Can you work these out from the model? Positions are in its coordinate system, mm. Coordinates: 2 decimals unless noted, no trailing zeros. Order: outer loops, then holes, each group sorted by start corner. A loop starts at its lowest first (then second) coordinate and runs counter-clockwise, first axis right, second up. Notation, with made-up numbers: (7, 73) -> (30, 73) arc R11 ccw to (30, 84) -> close; hole circle Ø1 at (-32, -36). An arc over 180 degrees is marked (long way). Return JSON: item names as keys, results as strings. Group by question number.
1) If we section it at A-A, the plane x = -105: Please give me the cut outline in (y, z), then the cut area to 3 significant figures.
2) If we section it at B-B, the plane z = 38.75: State how many separate pieces and enclosed holes the cut face has, then the cut area to 3 significant figures.
3) If I drill on probe 1 along Y at (x, z) = (-108.5, 38.5); probe 2 along X at (y, z) = (92.5, 37.75); probe 3 along X at (y, z) = (-4, 37.75), over which ranges is the centre line in solid material (lowest first)? Write a range as from..to.
4) For pin 1 (3.5 mm diameter, centred on x = -138.5, y = 71.5, fed in from +Z), with a flat end and sliding along its axis, tell me the tip position at first contact or that it passes through.
from build123d import *

# Parameters (mm, degrees)
SKETCH007_W     = 152.4
SKETCH007_H     = 127
PAD005_DEPTH    = 6.35
SKETCH085_R     = 2.2606
POCKET013_DEPTH = 6.351
SKETCH095_R     = 3.683
POCKET023_DEPTH = 4.318


with BuildPart() as part:
    # Sketch007 → Pad005 (new body)
    with BuildSketch(Plane.XY):
        Rectangle(SKETCH007_W, SKETCH007_H)
    extrude(amount=PAD005_DEPTH)

    # Sketch085 (on Face6 of Pad005) → Pocket013 (cut, through all)
    with BuildSketch(Plane.XY.offset(6.35)):
        with Locations((-38.1, 58.7375)):
            Circle(SKETCH085_R)
        with Locations((38.1, 58.7375)):
            Circle(SKETCH085_R)
        with Locations((71.4375, 38.1)):
            Circle(SKETCH085_R)
        with Locations((71.4375, -38.1)):
            Circle(SKETCH085_R)
        with Locations((38.1, -58.7375)):
            Circle(SKETCH085_R)
        with Locations((-38.1, -58.7375)):
            Circle(SKETCH085_R)
        with Locations((-71.4375, -38.1)):
            Circle(SKETCH085_R)
        with Locations((-71.4375, 38.1)):
            Circle(SKETCH085_R)
    extrude(amount=-POCKET013_DEPTH, mode=Mode.SUBTRACT)

    # Sketch095 (on Face6 of Pad005) → Pocket023 (cut)
    with BuildSketch(Plane.XY.offset(6.35)):
        with Locations((-38.1, 58.7375)):
            Circle(SKETCH095_R)
        with Locations((38.1, 58.7375)):
            Circle(SKETCH095_R)
        with Locations((71.4375, 38.1)):
            Circle(SKETCH095_R)
        with Locations((71.4375, -38.1)):
            Circle(SKETCH095_R)
        with Locations((38.1, -58.7375)):
            Circle(SKETCH095_R)
        with Locations((-38.1, -58.7375)):
            Circle(SKETCH095_R)
        with Locations((-71.4375, -38.1)):
            Circle(SKETCH095_R)
        with Locations((-71.4375, 38.1)):
            Circle(SKETCH095_R)
    extrude(amount=-POCKET023_DEPTH, mode=Mode.SUBTRACT)


with BuildPart() as part_1:
    # Body007 placement: moved
    add(part.part.moved(Location((-67.5132, 35.1028, 34.671))))


solid = part_1.part
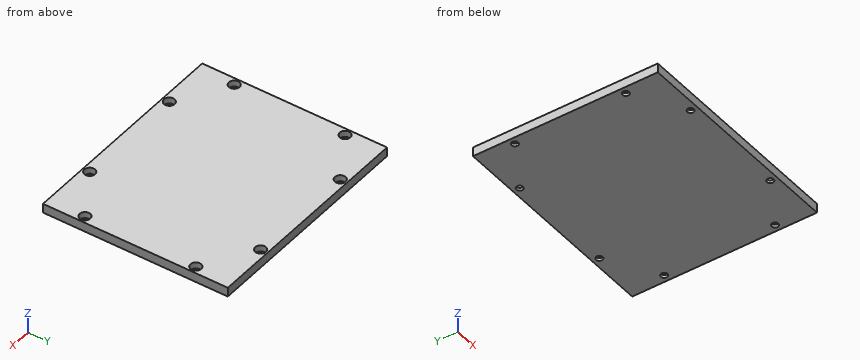
Result sheet:
{
 "1": {"outline": "(-28.4, 34.67) -> (-25.81, 34.67) -> (-25.81, 36.7) -> (-27.27, 36.7) -> (-27.27, 41.02) -> (-28.4, 41.02) -> close; (-21.46, 34.67) -> (91.66, 34.67) -> (91.66, 36.7) -> (90.21, 36.7) -> (90.21, 41.02) -> (-20, 41.02) -> (-20, 36.7) -> (-21.46, 36.7) -> close; (96.02, 34.67) -> (98.6, 34.67) -> (98.6, 41.02) -> (97.47, 41.02) -> (97.47, 36.7) -> (96.02, 36.7) -> close", "area": "726 mm2"},
 "2": {"separate pieces": "1", "enclosed holes": "8", "area": "19,000 mm2"},
 "3": {"probe 1": "y = -28.4..-25.92, -21.35..91.55, 96.13..98.6", "probe 2": "x = -143.71..-109.04, -102.18..-32.84, -25.98..8.69", "probe 3": "x = -143.71..-142.49, -135.41..0.38, 7.47..8.69"},
 "4": {"pin 1": "stops at z = 36.7"}
}
